Could you check a few things on this model? Use its own coordinates, in mm. Round coordinates to 2 decimals unless told otherwise and drop trailing zeros. Write each loop counter-clockwise with the first axis right and the second up, starting at its lowest first coordinate (ties: lowest second). Pieces come first, ordered by that corner, then holes. Notation, with made-up numbers: (-5.5, 40) -> (28.5, 40) arc R7 cw to (28.5, 51) -> close; hole circle Ø6 at (66.5, 8.25). An arc over 180 degrees is marked (long way). Answer as CSV lines item,"result". Start each with the question number.
Q1. If I drill on line 1 (Y direction, x = 0, z = 3.5); line 2 (X direction, y = 2, z = 5.5); line 3 (Y direction, x = -21, z = 5), over which ranges is the centre line in solid material (lowest first)? Write a range as [from, to].
Q2. Imagine slicing it at D-D on y = 40. Please give me the cut outline in (x, z).
Q3. Will these pins go through, and if not, where does the flat tip stop? pin 1 Ø4 at (y, z) = (10, 5.5) entering from +X; pin 2 Ø1.5 at (y, z) = (-8, 2.5) entering from +X; pin 3 Ø1 at (x, z) = (17.5, 8.5) entering from +Y.
Q4. Imagine slicing it at C-C on z = 4.75. Please give me the cut outline in (x, y), and give its area (3 significant figures).
Q5. Imagine slicing it at B-B on x = 0. Please give me the cut outline in (y, z), and give its area (3 significant figures).
Q6. Imagine slicing it at A-A on y = 0. Please give me the cut outline in (x, z), and give its area (3 significant figures).
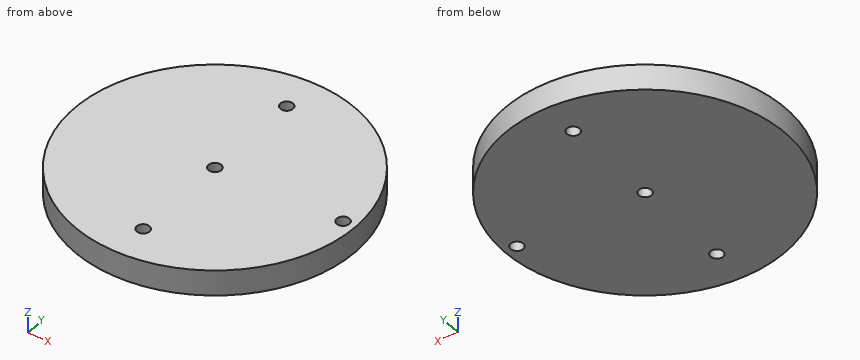
from build123d import *

# Parameters (mm, degrees)
SKETCH_1_R          = 55
EXTRUDE_1_DEPTH     = 10
SKETCH_2_R          = 2.5
CUT_EXTRUDE_1_DEPTH = 79.421935707
SKETCH_4_R          = 2.5
CUT_EXTRUDE_2_DEPTH = 79.421935707


with BuildPart() as part:
    # 草图1 → 凸台-拉伸1 (new body)
    with BuildSketch(Plane.XY):
        Circle(SKETCH_1_R)
    extrude(amount=EXTRUDE_1_DEPTH)

    # 草图2 → 切除-拉伸1 (cut, through all)
    with BuildSketch(Plane.XY.offset(10)):
        Circle(SKETCH_2_R)
        with Locations((50, 0)):
            Circle(SKETCH_2_R)
    extrude(amount=-CUT_EXTRUDE_1_DEPTH, mode=Mode.SUBTRACT)

    # 草图4 → 切除-拉伸2 (cut, through all)
    with BuildSketch(Plane(origin=(0, 0, 0), x_dir=(-1, 0, 0), z_dir=(0, 0, -1))):
        with Locations((0, -40)):
            Circle(SKETCH_4_R)
        with Locations((0, 40)):
            Circle(SKETCH_4_R)
    extrude(amount=-CUT_EXTRUDE_2_DEPTH, mode=Mode.SUBTRACT)


solid = part.part
Checks:
1,line 1,"[-55, -42.5], [-37.5, -2.5], [2.5, 37.5], [42.5, 55]"
1,line 2,"[-54.96, -1.5], [1.5, 48.5], [51.5, 54.96]"
1,line 3,"[-50.83, 50.83]"
2,outline,"(-37.75, 0) -> (-2.5, 0) -> (-2.5, 10) -> (-37.75, 10) -> close; (2.5, 0) -> (37.75, 0) -> (37.75, 10) -> (2.5, 10) -> close"
3,pin 1,"x = 54.42"
3,pin 2,"x = 54.52"
3,pin 3,"y = 52.31"
4,outline,"circle Ø110 at (0, 0); hole circle Ø5 at (0, -40); hole circle Ø5 at (0, 0); hole circle Ø5 at (0, 40); hole circle Ø5 at (50, 0)"
4,area,"9,420 mm^2"
5,outline,"(-55, 0) -> (-42.5, 0) -> (-42.5, 10) -> (-55, 10) -> close; (-37.5, 0) -> (-2.5, 0) -> (-2.5, 10) -> (-37.5, 10) -> close; (2.5, 0) -> (37.5, 0) -> (37.5, 10) -> (2.5, 10) -> close; (42.5, 0) -> (55, 0) -> (55, 10) -> (42.5, 10) -> close"
5,area,"950 mm^2"
6,outline,"(-55, 0) -> (-2.5, 0) -> (-2.5, 10) -> (-55, 10) -> close; (2.5, 0) -> (47.5, 0) -> (47.5, 10) -> (2.5, 10) -> close; (52.5, 0) -> (55, 0) -> (55, 10) -> (52.5, 10) -> close"
6,area,"1,000 mm^2"
